from build123d import *
from build123d.topology import SkipClean

# Parameters (mm, degrees)
SKETCH1_R           = 15
BOSS_EXTRUDE1_DEPTH = 2
CUT_EXTRUDE1_DEPTH  = 10


with BuildPart() as part:
    # Sketch1 → Boss-Extrude1 (new body)
    with BuildSketch(Plane.XY):
        Circle(SKETCH1_R)
        with BuildLine():
            ThreePointArc((-5.499090834, 5.1), (0, -7.5), (5.499090834, 5.1))
            Line((5.499090834, 5.1), (-5.499090834, 5.1))
        make_face(mode=Mode.SUBTRACT)
    extrude(amount=-BOSS_EXTRUDE1_DEPTH)

    # Sketch3 → Loft2 section 0
    with BuildSketch(Plane.XY, mode=Mode.PRIVATE) as loft2_s0:
        with BuildLine():
            Line((0, 47.4), (0, 43.9))
            ThreePointArc((0, 43.9), (5.730099838, 43.524429414), (11.36215608, 42.404143774))
            Line((11.36215608, 42.404143774), (12.268022738, 45.784884166))
            ThreePointArc((12.268022738, 45.784884166), (14.253454897, 45.206183465), (16.211754794, 44.541430225))
            Line((16.211754794, 44.541430225), (15.014684292, 41.252506053))
            ThreePointArc((15.014684292, 41.252506053), (20.270764121, 38.939775577), (25.180005556, 35.960774744))
            Line((25.180005556, 35.960774744), (27.187523083, 38.827806899))
            ThreePointArc((27.187523083, 38.827806899), (28.855291735, 37.60494833), (30.468132699, 36.310506604))
            Line((30.468132699, 36.310506604), (28.218376065, 33.629351053))
            ThreePointArc((28.218376065, 33.629351053), (32.366475086, 29.658410114), (35.960774744, 25.180005556))
            Line((35.960774744, 25.180005556), (38.827806899, 27.187523083))
            ThreePointArc((38.827806899, 27.187523083), (39.976754532, 25.468001436), (41.049604139, 23.7))
            Line((41.049604139, 23.7), (38.018515226, 21.95))
            ThreePointArc((38.018515226, 21.95), (40.558311477, 16.799802681), (42.404143774, 11.36215608))
            Line((42.404143774, 11.36215608), (45.784884166, 12.268022738))
            ThreePointArc((45.784884166, 12.268022738), (46.276430737, 10.259237701), (46.679887493, 8.230923621))
            Line((46.679887493, 8.230923621), (43.233060357, 7.623155))
            ThreePointArc((43.233060357, 7.623155), (43.858216927, 1.914891105), (43.732947246, -3.826137107))
            Line((43.732947246, -3.826137107), (47.21962869, -4.131182206))
            ThreePointArc((47.21962869, -4.131182206), (46.994486429, -6.186941511), (46.679887493, -8.230923621))
            Line((46.679887493, -8.230923621), (43.233060357, -7.623155))
            ThreePointArc((43.233060357, -7.623155), (41.868174138, -13.200984598), (39.786911851, -18.55294169))
            Line((39.786911851, -18.55294169), (42.958989106, -20.032105607))
            ThreePointArc((42.958989106, -20.032105607), (42.044313493, -21.886884267), (41.049604139, -23.7))
            Line((41.049604139, -23.7), (38.018515226, -21.95))
            ThreePointArc((38.018515226, -21.95), (34.828211639, -26.724626733), (31.041987694, -31.041987694))
            Line((31.041987694, -31.041987694), (33.516861428, -33.516861428))
            ThreePointArc((33.516861428, -33.516861428), (32.022975841, -34.946945765), (30.468132699, -36.310506604))
            Line((30.468132699, -36.310506604), (28.218376065, -33.629351053))
            ThreePointArc((28.218376065, -33.629351053), (23.587452806, -37.024884471), (18.55294169, -39.786911851))
            Line((18.55294169, -39.786911851), (20.032105607, -42.958989106))
            ThreePointArc((20.032105607, -42.958989106), (18.139194694, -43.791889841), (16.211754794, -44.541430225))
            Line((16.211754794, -44.541430225), (15.014684292, -41.252506053))
            ThreePointArc((15.014684292, -41.252506053), (9.501699052, -42.859394713), (3.826137107, -43.732947246))
            Line((3.826137107, -43.732947246), (4.131182206, -47.21962869))
            ThreePointArc((4.131182206, -47.21962869), (2.067558961, -47.354885703), (0, -47.4))
            Line((0, -47.4), (0, -43.9))
            ThreePointArc((0, -43.9), (-5.730099838, -43.524429414), (-11.36215608, -42.404143774))
            Line((-11.36215608, -42.404143774), (-12.268022738, -45.784884166))
            ThreePointArc((-12.268022738, -45.784884166), (-14.253454897, -45.206183465), (-16.211754794, -44.541430225))
            Line((-16.211754794, -44.541430225), (-15.014684292, -41.252506053))
            ThreePointArc((-15.014684292, -41.252506053), (-20.270764121, -38.939775577), (-25.180005556, -35.960774744))
            Line((-25.180005556, -35.960774744), (-27.187523083, -38.827806899))
            ThreePointArc((-27.187523083, -38.827806899), (-28.855291735, -37.60494833), (-30.468132699, -36.310506604))
            Line((-30.468132699, -36.310506604), (-28.218376065, -33.629351053))
            ThreePointArc((-28.218376065, -33.629351053), (-32.366475086, -29.658410114), (-35.960774744, -25.180005556))
            Line((-35.960774744, -25.180005556), (-38.827806899, -27.187523083))
            ThreePointArc((-38.827806899, -27.187523083), (-39.976754532, -25.468001436), (-41.049604139, -23.7))
            Line((-41.049604139, -23.7), (-38.018515226, -21.95))
            ThreePointArc((-38.018515226, -21.95), (-40.558311477, -16.799802681), (-42.404143774, -11.36215608))
            Line((-42.404143774, -11.36215608), (-45.784884166, -12.268022738))
            ThreePointArc((-45.784884166, -12.268022738), (-46.276430737, -10.259237701), (-46.679887493, -8.230923621))
            Line((-46.679887493, -8.230923621), (-43.233060357, -7.623155))
            ThreePointArc((-43.233060357, -7.623155), (-43.858216927, -1.914891105), (-43.732947246, 3.826137107))
            Line((-43.732947246, 3.826137107), (-47.21962869, 4.131182206))
            ThreePointArc((-47.21962869, 4.131182206), (-46.994486429, 6.186941511), (-46.679887493, 8.230923621))
            Line((-46.679887493, 8.230923621), (-43.233060357, 7.623155))
            ThreePointArc((-43.233060357, 7.623155), (-41.868174138, 13.200984598), (-39.786911851, 18.55294169))
            Line((-39.786911851, 18.55294169), (-42.958989106, 20.032105607))
            ThreePointArc((-42.958989106, 20.032105607), (-42.044313493, 21.886884267), (-41.049604139, 23.7))
            Line((-41.049604139, 23.7), (-38.018515226, 21.95))
            ThreePointArc((-38.018515226, 21.95), (-34.828211639, 26.724626733), (-31.041987694, 31.041987694))
            Line((-31.041987694, 31.041987694), (-33.516861428, 33.516861428))
            ThreePointArc((-33.516861428, 33.516861428), (-32.022975841, 34.946945765), (-30.468132699, 36.310506604))
            Line((-30.468132699, 36.310506604), (-28.218376065, 33.629351053))
            ThreePointArc((-28.218376065, 33.629351053), (-23.587452806, 37.024884471), (-18.55294169, 39.786911851))
            Line((-18.55294169, 39.786911851), (-20.032105607, 42.958989106))
            ThreePointArc((-20.032105607, 42.958989106), (-18.139194694, 43.791889841), (-16.211754794, 44.541430225))
            Line((-16.211754794, 44.541430225), (-15.014684292, 41.252506053))
            ThreePointArc((-15.014684292, 41.252506053), (-9.501699052, 42.859394713), (-3.826137107, 43.732947246))
            Line((-3.826137107, 43.732947246), (-4.131182206, 47.21962869))
            ThreePointArc((-4.131182206, 47.21962869), (-2.067558961, 47.354885703), (0, 47.4))
        make_face()
    loft([loft2_s0.sketch, Vertex(0, 0, 100)])

    # Sketch1_4 → Cut-Extrude1 (cut)
    with SkipClean():  # the faces are left unmerged after this step: merging them gives an invalid solid
        with BuildSketch(Plane.XY):
            with BuildLine():
                Line((-5.499090834, 5.1), (5.499090834, 5.1))
                ThreePointArc((5.499090834, 5.1), (0, -7.5), (-5.499090834, 5.1))
            make_face()
        extrude(amount=CUT_EXTRUDE1_DEPTH, mode=Mode.SUBTRACT)


solid = part.part
Can you work these out from the model? Positions are in its coordinate system, mm. A direction names the side the tool comes from. Give positions to 0.01 mm unless a question says otherwise; leave off trailing zeros. One line per question, with ' | ' between items.
Item 1: We'd pull the mould along Y, two halves only. Please class faces 6 (the face through (0, -34, 24)), 7 (the face through (30.926, -14.421, 24.307)), 8 (the face through (-24, 24, 24)), 9 (the face through (-29.74, 17.17, 24.31)): released by +Y, released by -Y, zero draft, split by the parting line, or undercut.
Answer block:
face 6: zero draft | face 7: undercut | face 8: undercut | face 9: released by +Y
Item 2: Please list where these lines run through material, in increasing order: L1, parallel to Z at x = 40, y = 11; L2, parallel to X at y = 18, z = 49; L3, parallel to Y at x = 19, z = 53.
Answer block:
L1: z = 0 to 5.5 | L2: x = -16.14 to -15.1, -13.31 to 15.1 | L3: y = -10.97 to -8.86, -8.04 to 8.04, 10.97 to 11.63
Item 3: I'm going to push flat-ended pins straight in: pin 1 Ø1.5 at (x, z) = (7.5, 71) entering from -Y; pin 2 Ø0.6 at (x, z) = (1.5, -1.5) entering from -Y; pin 3 Ø1.5 at (y, z) = (4, 74.5) entering from -X; pin 4 Ø14 at (y, z) = (-28.5, 69.5) entering from -X. Where does each tip first touch, or does it pass through?
Answer block:
pin 1: stops at y = -10.93 | pin 2: stops at y = -14.95 | pin 3: stops at x = -10.89 | pin 4: passes through
Item 4: For faces 1 (the face through (2.974, -33.993, 24.307)), 2 (the face through (11.746, 32.273, 24.307)), 3 (the face through (32.96, 8.83, 24.31)), 4 (the face through (11.746, -32.273, 24.307)), 5 (the face through (11, -11, 0)), which set-ups out of +Z, -Z, +X, -X, +Y, -Y let a thin tool reach every point of the face, with its end or its side?
Answer block:
face 1: +Z | face 2: +Z, +X | face 3: +Z, +Y | face 4: +Z, -Y | face 5: -Z
